Part print with two shaded views. Sizes in mm from the minimum x, y, z corner. A direction names the side the tool comes from. Give positions to 0.01 mm unless a question says otherwise; leave off trailing zeros. Order: outer loops, then holes, each group sorted by start corner. A loop starts at its lowest first (then second) coordinate and runs counter-clockwise, first axis right, second up. Notation, with made-up numbers: (24, -36.5) -> (28, -36.5) arc R15 ccw to (28, -26.5) -> close; hole circle Ø4 at (-25.75, 1.25). An arc over 180 degrees is marked (long way). Answer as CSV lines item,"result".
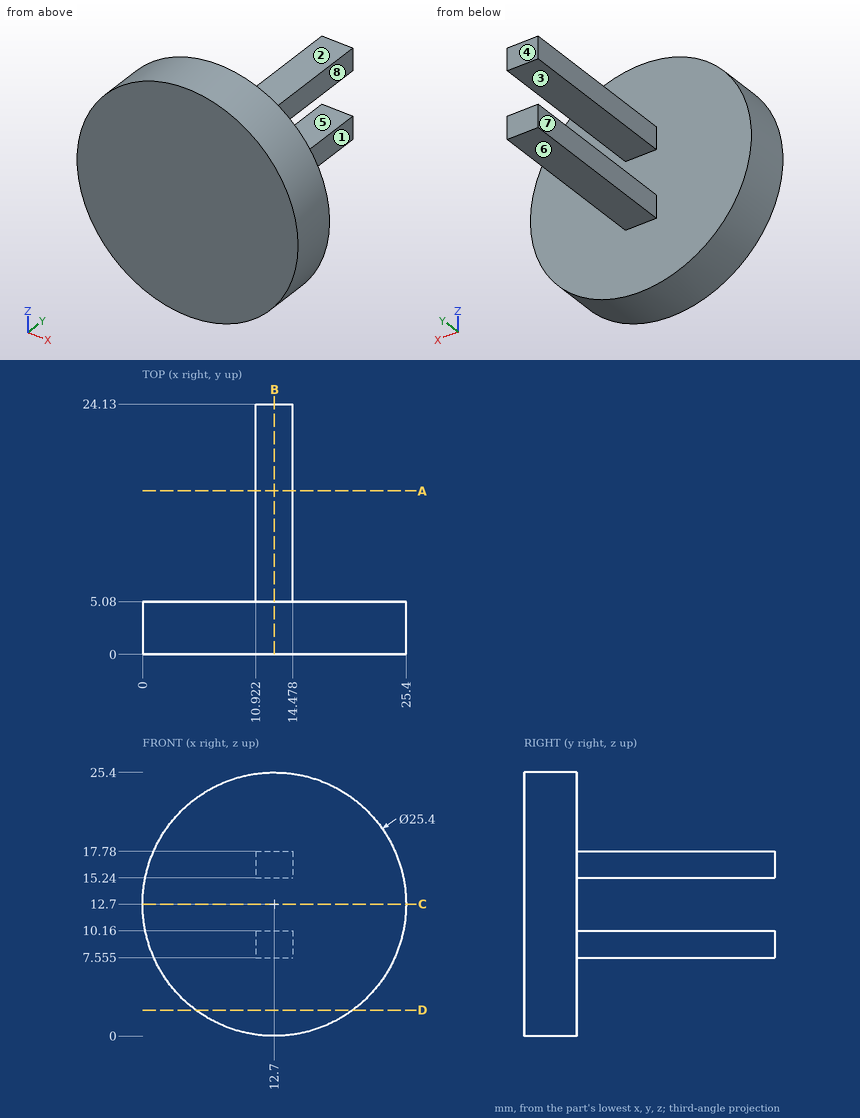
1) Band-saw the part on D-D, the plane z = 2.5. Write the cut outline in (x, y).
Data:
outline,"(5.13, 0) -> (20.27, 0) -> (20.27, 5.08) -> (5.13, 5.08) -> close"
2) Band-saw the part on A-A, the plane y = 15.75. Write the cut outline in (x, z) (1 decimal).
Data:
outline,"(10.9, 7.6) -> (14.5, 7.6) -> (14.5, 10.2) -> (10.9, 10.2) -> close; (10.9, 15.2) -> (14.5, 15.2) -> (14.5, 17.8) -> (10.9, 17.8) -> close"
3) Which spindle directions (+Z, -Z, +X, -X, +Y, -Y) get a long thin tool onto all of the face, cutting with end or side? Do the marked faces 4, 5, 6, 7 and 8. Say none if no direction does.
Data:
face 4,"+Z, -Z, +X, -X, +Y"
face 5,"+X, -X, +Y"
face 6,"-Z, +X, -X, +Y"
face 7,"+Z, -Z, -X, +Y"
face 8,"+Z, -Z, +X, +Y"
4) Wall check: line 1 along Y through (x, z) = (17, 21.5); line 2 along Z through (x, y) = (14, 23) (1 decimal); line 3 along X through (y, z) = (17.5, 8). Give the ranges that are in metal, low to high. Write a range as [from, to].
Data:
line 1,"y = [0, 5.08]"
line 2,"z = [7.6, 10.2], [15.2, 17.8]"
line 3,"x = [10.92, 14.48]"
5) Pin check, flat tips, straight feed: P1, Ø6, axis at x = 5.5, z = 3.5, coming from the +Y side; P2, Ø2, axis at y = 10.5, z = 17, coming from the +X side; P3, Ø3, axis at x = 13.5, y = 14.5, coming from the -Z side (1 decimal). Stop position of each tip, or through.
Data:
P1,"stops at y = 5.08"
P2,"stops at x = 14.48"
P3,"stops at z = 7.6"
6) Band-saw the part on C-C, the plane z = 12.7. Write the cut outline in (x, y), then the cut area to 3 significant figures.
Data:
outline,"(0, 0) -> (25.4, 0) -> (25.4, 5.08) -> (0, 5.08) -> close"
area,"129 mm2"
7) Band-saw the part on B-B, the plane x = 12.7. Write the cut outline in (y, z) (1 decimal), then the cut area to 3 significant figures.
Data:
outline,"(0, 0) -> (5.1, 0) -> (5.1, 7.6) -> (24.1, 7.6) -> (24.1, 10.2) -> (5.1, 10.2) -> (5.1, 15.2) -> (24.1, 15.2) -> (24.1, 17.8) -> (5.1, 17.8) -> (5.1, 25.4) -> (0, 25.4) -> close"
area,"227 mm2"
8) Pull direction Z, two halves, no side cores. Call the marked faces 1, 2 and 3: pulls with the +Z half, pulls with the -Z half, needs draft (parallel to the pull), parting line crosses it, or undercut.
Data:
face 1,"needs draft"
face 2,"pulls with the +Z half"
face 3,"undercut"
